```python
from build123d import *

# Parameters (mm, degrees)
ESQUISSE1_W                = 45
ESQUISSE1_H                = 15
BOSS_EXTRU_1_DEPTH         = 0.5
BOSS_EXTRU_2_DEPTH         = 15
ESQUISSE3_W                = 33.5
ESQUISSE3_H                = 7.5
ENL_V_MAT_EXTRU_1_DEPTH    = 48.647140523
BOSS_EXTRU_5_DEPTH         = 20
BOSS_EXTRU_5_DEPTH_BACK    = 20
ESQUISSE10_W               = 64.680470467
ESQUISSE10_H               = 24.042247858
ENL_V_MAT_EXTRU_3_DEPTH    = 3
ESQUISSE11_W               = 33.5
ESQUISSE11_H               = 0.5
ENL_V_MAT_EXTRU_4_DEPTH    = 47.840153715
ESQUISSE12_W               = 10.593660794
ESQUISSE12_H               = 24.624800323
ENL_V_MAT_EXTRU_5_DEPTH    = 0.5
BOSS_EXTRU_6_DEPTH         = 12
BOSS_EXTRU_7_DEPTH         = 83
BOSS_EXTRU_7_DEPTH_BACK    = 12
ESQUISSE13_3_W             = 3
ESQUISSE13_3_H             = 5
ENL_V_MAT_EXTRU_6_DEPTH    = 185
R_P_TITION_LIN_AIRE2_COUNT = 63
R_P_TITION_LIN_AIRE2_PITCH = 1.5
ESQUISSE8_W                = 33.5
ESQUISSE8_H                = 3
ENL_V_MAT_EXTRU_2_DEPTH    = 0.5


with BuildPart() as part:
    # Esquisse1 → Boss.-Extru.1 (new body)
    with BuildSketch(Plane.XY):
        with Locations((22.5, 7.5)):
            Rectangle(ESQUISSE1_W, ESQUISSE1_H)
    extrude(amount=BOSS_EXTRU_1_DEPTH)

    # Esquisse2 → Boss.-Extru.2 (add)
    with BuildSketch(Plane(origin=(0, 15, 0), x_dir=(1, 0, 0), z_dir=(0, 1, 0))):
        with BuildLine():
            ThreePointArc((0.5, -0.5), (2.5, -2.5), (0.5, -4.5))
            Line((0.5, -4.5), (0, -4.5))
            Line((0, -4.5), (0, -5))
            Line((0, -5), (0.5, -5))
            Line((0.5, -5), (2, -5))
            Line((2, -5), (5.75, -0.5))
            Line((5.75, -0.5), (0.5, -0.5))
        make_face()
        with BuildLine():
            Line((44.5, -0.5), (39.25, -0.5))
            Line((39.25, -0.5), (43, -5))
            Line((43, -5), (44.5, -5))
            Line((44.5, -5), (45, -5))
            Line((45, -5), (45, -4.5))
            Line((45, -4.5), (44.5, -4.5))
            ThreePointArc((44.5, -4.5), (42.5, -2.5), (44.5, -0.5))
        make_face()
    extrude(amount=-BOSS_EXTRU_2_DEPTH)

    # Esquisse3 → Enlèv. mat.-Extru.1 (cut, through all)
    with BuildSketch(Plane.XY.offset(0.5)):
        with Locations((22.5, 3.75)):
            Rectangle(ESQUISSE3_W, ESQUISSE3_H)
    extrude(amount=-ENL_V_MAT_EXTRU_1_DEPTH, mode=Mode.SUBTRACT)

    # Esquisse7 → Boss.-Extru.5 (add, two sides: drawn at the far end of the back side and taken through both)
    with BuildSketch(Plane.ZY.offset(-22.5).offset(-BOSS_EXTRU_5_DEPTH_BACK)):
        with BuildLine():
            Line((1, 7.5), (2, 7.5))
            Line((2, 7.5), (2, 14.625))
            ThreePointArc((2, 14.625), (1.625, 15), (1.25, 14.625))
            Line((1.25, 14.625), (1, 7.5))
        make_face()
    extrude(amount=BOSS_EXTRU_5_DEPTH + BOSS_EXTRU_5_DEPTH_BACK)

    # Esquisse10 → Enlèv. mat.-Extru.3 (cut)
    with BuildSketch(Plane.XZ):
        with Locations((25.714759003, 2.202104928)):
            Rectangle(ESQUISSE10_W, ESQUISSE10_H)
    extrude(amount=-ENL_V_MAT_EXTRU_3_DEPTH, mode=Mode.SUBTRACT)

    # Esquisse11 → Enlèv. mat.-Extru.4 (cut, through all)
    with BuildSketch(Plane(origin=(0, 15, 0), x_dir=(1, 0, 0), z_dir=(0, 1, 0))):
        with Locations((22.5, -0.25)):
            Rectangle(ESQUISSE11_W, ESQUISSE11_H)
    extrude(amount=-ENL_V_MAT_EXTRU_4_DEPTH, mode=Mode.SUBTRACT)

    # Esquisse12 → Enlèv. mat.-Extru.5 (cut)
    with BuildSketch(Plane.ZY):
        with Locations((2.946764515, 5.852855815)):
            Rectangle(ESQUISSE12_W, ESQUISSE12_H)
    extrude(amount=-ENL_V_MAT_EXTRU_5_DEPTH, mode=Mode.SUBTRACT)

    # Esquisse13 → Boss.-Extru.6 (add)
    with BuildSketch(Plane(origin=(0, 15, 0), x_dir=(1, 0, 0), z_dir=(0, 1, 0))):
        with BuildLine():
            Line((-2, -5), (0.5, -5))
            Line((0.5, -5), (0.5, -4.5))
            ThreePointArc((0.5, -4.5), (-1.5, -2.5), (0.5, -0.5))
            Line((0.5, -0.5), (0.5, 0))
            Line((0.5, 0), (-2, 0))
            Line((-2, 0), (-2, -5))
        make_face()
    extrude(amount=-BOSS_EXTRU_6_DEPTH)

    # Esquisse13<3> → Boss.-Extru.7 (add, two sides: drawn at the far end of the back side and taken through both)
    with BuildSketch(Plane(origin=(0, 15, 0), x_dir=(1, 0, 0), z_dir=(0, 1, 0)).offset(-BOSS_EXTRU_7_DEPTH_BACK)):
        with Locations((-3.5, -2.5)):
            Rectangle(ESQUISSE13_3_W, ESQUISSE13_3_H)
    extrude(amount=BOSS_EXTRU_7_DEPTH + BOSS_EXTRU_7_DEPTH_BACK)

    # Esquisse14 → Enlèv. mat.-Extru.6 (cut)
    with BuildSketch(Plane(origin=(0, 0, 0), x_dir=(-1, 0, 0), z_dir=(0, 0, -1))):
        Polygon((5, 98), (4.250024873, 97.243891844), (5, 96.5), align=None)
    enl_v_mat_extru_6 = extrude(amount=-ENL_V_MAT_EXTRU_6_DEPTH, mode=Mode.SUBTRACT)

    # Répétition linéaire2: Enlèv. mat.-Extru.6 ×63
    with Locations(*[(0, -i * R_P_TITION_LIN_AIRE2_PITCH, 0) for i in range(1, R_P_TITION_LIN_AIRE2_COUNT)]):
        add(enl_v_mat_extru_6, mode=Mode.SUBTRACT)

    # Esquisse8 → Enlèv. mat.-Extru.2 (cut)
    with BuildSketch(Plane(origin=(0, 0, 0), x_dir=(-1, 0, 0), z_dir=(0, 0, -1))):
        with Locations((-22.5, 9)):
            Rectangle(ESQUISSE8_W, ESQUISSE8_H)
    extrude(amount=-ENL_V_MAT_EXTRU_2_DEPTH, mode=Mode.SUBTRACT)


solid = part.part
```
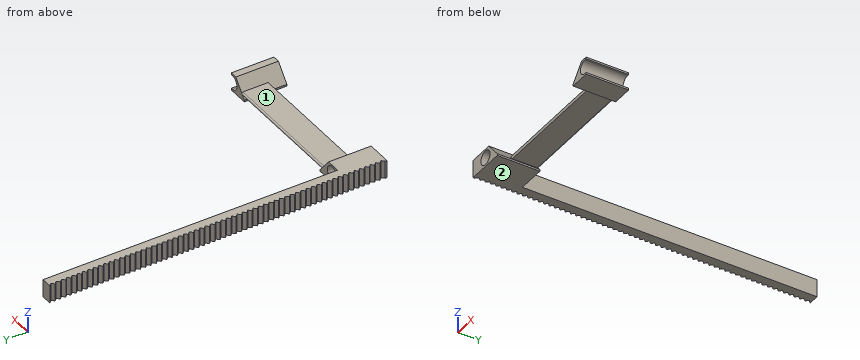
Could you check a few things on this model? Use its own coordinates, in mm. Face numbers are marked on the shaded views. Give positions to 0.01 mm unless a question says otherwise; leave off trailing zeros. Order: outer loops, then holes, each group sorted by start corner. A loop starts at its lowest first (then second) coordinate and runs counter-clockwise, first axis right, second up.
Q1. Suppose I cut it at C-C, the plane x = 17.5. Write out the boundary of the cut face in (y, z) (3 decimals).
Q2. Suppose I cut it at A-A, the plane x = 0.5. Write out the boundary of the cut face in (y, z).
Q3. Suppose I cut it at B-B, the plane z = 3.7. Count the separate pieces of the cut face and the enclosed holes in it, and give its area (3 significant figures).
Q4. We'd pull the mould along X, two halves only. Please class the marked faces 1 and 2: +X half, -X half, draft (parallel to the pull), parting line (faces both ways), or undercut.
Q5. If I drill on line 1 along X through (y, z) = (9.25, 2.5); line 2 along X through (y, z) = (10.5, 2.5); line 3 along Z through (x, y) = (17, 8), over which ranges is the centre line in solid material (lowest first)?
Q6. I'm going to push flat-ended pins straight in: P1, Ø1, axis at x = 23.5, z = 1.5, coming from the -Y side; P2, Ø2, axis at y = 40.5, z = 0.5, coming from the +X side; P3, Ø2, axis at x = 24.5, y = 9.5, coming from the +Z side. Where does each tip first touch, or does it pass through?
Solution:
1. outline: (7.5, 1) - (14.625, 1.25) arc R0.375 ccw to (14.625, 2) - (7.5, 2) - close
2. outline: (3, 0) - (15, 0) - (15, 0.5) - (3, 0.5) - close; (3, 4.5) - (15, 4.5) - (15, 5) - (3, 5) - close
3. separate pieces: 3
3. enclosed holes: 0
3. area: 284 mm2
4. face 1: undercut
4. face 2: draft
5. line 1: x = -4.75 to -1.5, 2.5 to 4.08, 40.92 to 42.5
5. line 2: x = -4.5 to -1.5, 2.5 to 4.08, 40.92 to 42.5
5. line 3: z = 1.02 to 2
6. P1: stops at y = 7.5
6. P2: stops at x = -2
6. P3: stops at z = 2
